Work out the finished part from the listing and answer in its coordinate system (mm). Face numbers are marked on the shaded views. A direction names the side the tool comes from. Give positions to 0.01 mm unless a question says otherwise; leave off trailing zeros. Loops run counter-clockwise (first coordinate to the right, second up) from the corner with the lowest first, then second, coordinate; pieces in that order, holes last.
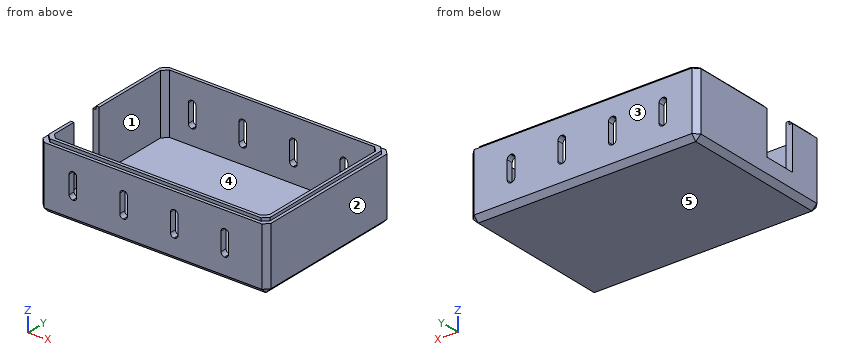
```python
from build123d import *

# Parameters (mm, degrees)
F0_W      = 114.3
F0_H      = 78.74
F1_DEPTH  = 3.175
F2_W      = 114.3
F2_H      = 78.74
F2_W_2    = 107.95
F2_H_2    = 72.39
F3_DEPTH  = 28.575
F4_W      = 16.002
F4_H      = 21.844
F5_DEPTH  = 3.175
F7_DEPTH  = 1.5494
F8_SIZE   = 2.54
F9_SIZE   = 2.54
F10_SIZE  = 2.54
F11_W     = 3.81
F11_H     = 12.7
F12_DEPTH = 78.741
F13_R     = 1.778


with BuildPart() as f1:
    # F0 (on Top) → F1 (new body)
    with BuildSketch(Plane.XY):
        Rectangle(F0_W, F0_H)
    extrude(amount=F1_DEPTH)

    # F2 (on face) → F3 (join)
    with BuildSketch(Plane.XY.offset(3.175)):
        Rectangle(F2_W, F2_H)
        Rectangle(F2_W_2, F2_H_2, mode=Mode.SUBTRACT)
    extrude(amount=F3_DEPTH)

    # F4 (on face) → F5 (cut, through all)
    with BuildSketch(Plane(origin=(-57.15, 0, 0), x_dir=(0, -1, 0), z_dir=(-1, 0, 0))):
        with Locations((13.2334, 20.828)):
            Rectangle(F4_W, F4_H)
    extrude(amount=-F5_DEPTH, mode=Mode.SUBTRACT)

    # F6 (on face) → F7 (join)
    with BuildSketch(Plane.XY.offset(31.75)):
        Polygon((55.5498, 37.7698), (-55.5498, 37.7698), (-55.5498, -5.2324), (-53.975, -5.2324), (-53.975, 36.195), (53.975, 36.195), (53.975, -36.195), (-53.975, -36.195), (-53.975, -21.2344), (-55.5498, -21.2344), (-55.5498, -37.7698), (55.5498, -37.7698), align=None)
    extrude(amount=F7_DEPTH)

    # F8
    f8_edges = [f1.edges().sort_by_distance(p)[0] for p in [
        (57.15, 39.37, 15.875),
        (57.15, -39.37, 15.875),
        (-57.15, -39.37, 15.875),
        (-57.15, 39.37, 15.875),
        (0, 39.37, 0),
        (-57.15, 0, 0),
        (0, -39.37, 0),
        (57.15, 0, 0),
    ]]
    chamfer(f8_edges, length=F8_SIZE)

    # F9
    f9_edges = [f1.edges().sort_by_distance(p)[0] for p in [
        (-53.975, 36.195, 18.2372),
        (53.975, 36.195, 18.2372),
        (53.975, -36.195, 18.2372),
        (-53.975, -36.195, 18.2372),
    ]]
    chamfer(f9_edges, length=F9_SIZE)

    # F10
    f10_edges = [f1.edges().sort_by_distance(p)[0] for p in [
        (55.5498, 37.7698, 32.5247),
        (-55.5498, 37.7698, 32.5247),
        (-55.5498, -37.7698, 32.5247),
        (55.5498, -37.7698, 32.5247),
    ]]
    chamfer(f10_edges, length=F10_SIZE)

    # F11 (on face) → F12 (cut, through all)
    with BuildSketch(Plane.XZ.offset(39.37)):
        with Locations((-40.132, 17.145)):
            Rectangle(F11_W, F11_H)
        with Locations((-14.732, 17.145)):
            Rectangle(F11_W, F11_H)
        with Locations((10.668, 17.145)):
            Rectangle(F11_W, F11_H)
        with Locations((36.068, 17.145)):
            Rectangle(F11_W, F11_H)
    extrude(amount=-F12_DEPTH, mode=Mode.SUBTRACT)

    # F13
    f13_edges = [f1.edges().sort_by_distance(p)[0] for p in [
        (-42.037, -37.7825, 23.495),
        (-16.637, -37.7825, 23.495),
        (8.763, -37.7825, 23.495),
        (34.163, -37.7825, 23.495),
        (-38.227, -37.7825, 23.495),
        (-12.827, -37.7825, 23.495),
        (12.573, -37.7825, 23.495),
        (37.973, -37.7825, 23.495),
        (-42.037, -37.7825, 10.795),
        (-16.637, -37.7825, 10.795),
        (8.763, -37.7825, 10.795),
        (34.163, -37.7825, 10.795),
        (-38.227, -37.7825, 10.795),
        (-12.827, -37.7825, 10.795),
        (12.573, -37.7825, 10.795),
        (37.973, -37.7825, 10.795),
        (37.973, 37.7825, 23.495),
        (12.573, 37.7825, 23.495),
        (-12.827, 37.7825, 23.495),
        (-38.227, 37.7825, 23.495),
        (34.163, 37.7825, 23.495),
        (8.763, 37.7825, 23.495),
        (-16.637, 37.7825, 23.495),
        (-42.037, 37.7825, 23.495),
        (34.163, 37.7825, 10.795),
        (8.763, 37.7825, 10.795),
        (-16.637, 37.7825, 10.795),
        (-42.037, 37.7825, 10.795),
        (-38.227, 37.7825, 10.795),
        (-12.827, 37.7825, 10.795),
        (12.573, 37.7825, 10.795),
        (37.973, 37.7825, 10.795),
    ]]
    fillet(f13_edges, radius=F13_R)


solid = f1.part
```
Q1. Section C-C on y = 8.5 is taken. Give the vertices of the cut face in (x, z) (3 decimals).
Q2. Consider line 1 along X through (y, z) = (4, 21.5) (3 decimals); line 2 along Y through (x, z) = (15.5, 14) (3 decimals). Determine where each line is inside the solid, lowest interval first.
Q3. Section B-B on z = 28.5 is taken. Give the vertices of the cut face in (x, y) (3 decimals).
Q4. Section A-A on x = 20 is taken. Give the vertices of the cut face in (y, z) (3 decimals).
Q5. Section D-D on z = 20 is taken. State how many separate pieces and enclosed holes the cut face has, plus the area to 3 significant figures.
Q6. Determine the mould class of the marked faces 1, 2 and 3 for opening direction Y: +Y half, -Y half, draft (parallel to the pull), parting line (faces both ways), or undercut.
Q7. Which of the six approach directions +Z, -Z, +X, -X, +Y, -Y give full straight-line access (tool end or side, diameter ignored) to the marked faces 4 and 5?
Q8. Given pin 1 (5 mm diameter, centred on x = -15.5, y = -23, fed in from +Z) (3 decimals); pin 2 (1.6 mm diameter, centred on y = 38, z = 15.5, fed in from -X); pin 3 (1 mm diameter, centred on y = 37, z = 17.5, fed in from +X); pin 4 (0.8 mm diameter, centred on x = 0.5, z = 32.5, fed in from -Y), each flat-ended and moving along its own axis, determine where each tip first touches the part or whether it passes through.
Check result:
1. outline: (-57.15, 2.54) - (-54.61, 0) - (54.61, 0) - (57.15, 2.54) - (57.15, 31.75) - (55.55, 31.75) - (55.55, 33.299) - (53.975, 33.299) - (53.975, 3.175) - (-53.975, 3.175) - (-53.975, 33.299) - (-55.55, 33.299) - (-55.55, 31.75) - (-57.15, 31.75) - close
2. line 1: x = -57.15 to -53.975, 53.975 to 57.15
2. line 2: y = -39.37 to -36.195, 36.195 to 39.37
3. outline: (-57.15, -36.83) - (-54.61, -39.37) - (54.61, -39.37) - (57.15, -36.83) - (57.15, 36.83) - (54.61, 39.37) - (-54.61, 39.37) - (-57.15, 36.83) - (-57.15, -5.232) - (-53.975, -5.232) - (-53.975, 33.655) - (-51.435, 36.195) - (51.435, 36.195) - (53.975, 33.655) - (53.975, -33.655) - (51.435, -36.195) - (-51.435, -36.195) - (-53.975, -33.655) - (-53.975, -21.234) - (-57.15, -21.234) - close
4. outline: (-39.37, 2.54) - (-36.83, 0) - (36.83, 0) - (39.37, 2.54) - (39.37, 31.75) - (37.77, 31.75) - (37.77, 33.299) - (36.195, 33.299) - (36.195, 3.175) - (-36.195, 3.175) - (-36.195, 33.299) - (-37.77, 33.299) - (-37.77, 31.75) - (-39.37, 31.75) - close
5. separate pieces: 9
5. enclosed holes: 0
5. area: 1,040 mm2
6. face 1: undercut
6. face 2: draft
6. face 3: +Y half
7. face 4: +Z
7. face 5: -Z, +X, -X, +Y, -Y
8. pin 1: stops at z = 3.175
8. pin 2: stops at x = -56.78
8. pin 3: stops at x = 57.15
8. pin 4: stops at y = -37.77
